Source: CAD feature listing. Evaluate the final solid. Frame: model axes, mm. Face numbers are marked on the shaded views. Coordinates: 2 decimals unless noted, no trailing zeros. Loops run counter-clockwise (first coordinate to the right, second up) from the corner with the lowest first, then second, coordinate; pieces in that order, holes last. Notation, with made-up numbers: (-24.5, 32) -> (30.5, 32) arc R16 cw to (30.5, 62) -> close; hole circle Ø6 at (30.5, -20). An arc over 180 degrees is marked (long way). One line per question, with ' | ' between items. Start each with the question number.
```python
from build123d import *

# Parameters (mm, degrees)
ESQUISSE1_R             = 11
BOSS_EXTRU_1_DEPTH      = 20
ESQUISSE2_R             = 2
ENL_V_MAT_EXTRU_1_DEPTH = 163.249807396


with BuildPart() as part:
    # Esquisse1 → Boss.-Extru.1 (new body)
    with BuildSketch(Plane.XY):
        with BuildLine():
            Line((0, 0), (95, 0))
            Line((95, 0), (74, 108))
            ThreePointArc((74, 108), (47.5, 130), (21, 108))
            Line((21, 108), (0, 0))
        make_face()
        with Locations((47.5, 103.039772727)):
            Circle(ESQUISSE1_R, mode=Mode.SUBTRACT)
    extrude(amount=BOSS_EXTRU_1_DEPTH)

    # Esquisse2 → Enlèv. mat.-Extru.1 (cut, through all)
    with BuildSketch(Plane.XY.offset(20)):
        with Locations((63, 11)):
            Circle(ESQUISSE2_R)
        with Locations((32, 11)):
            Circle(ESQUISSE2_R)
        with Locations((32, 42)):
            Circle(ESQUISSE2_R)
        with Locations((63, 42)):
            Circle(ESQUISSE2_R)
    extrude(amount=-ENL_V_MAT_EXTRU_1_DEPTH, mode=Mode.SUBTRACT)


solid = part.part
```
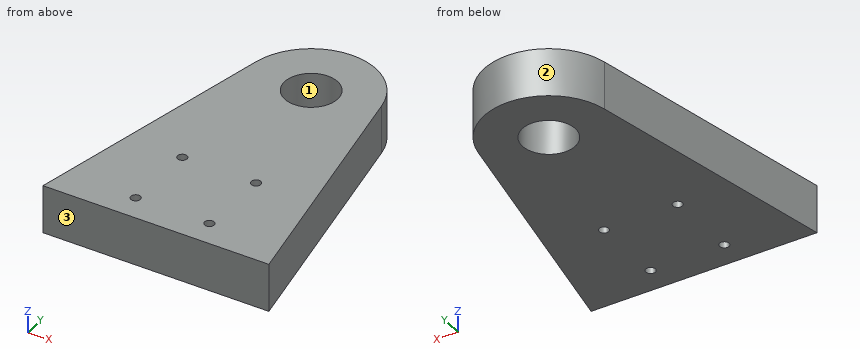
(1) Cut plane D-D, the plane x = 56.5. Return the cut outline in (y, z), and give its area (3 significant figures).
(2) Draft query along Y for the marked faces 1, 2 and 3. Return one class per face: pulls with the +Y half, pulls with the -Y half, needs draft (parallel to the pull), parting line crosses it, or undercut.
(3) Cut plane A-A, the plane y = 42. Return the cut outline in (x, z).
(4) Ray query, L1, parallel to Y at x = 47.5, z = 12; L2, parallel to Y at x = 32, z = 14.5; L3, parallel to X at y = 43.5, z = 1. Return the intervals inside material, ascending.
(5) Cut plane C-C, the plane z = 4. Return the cut outline in (x, y), and give its area (3 significant figures).
(6) Contact query for flat-ended pins moving along their axis: pin 1 Ø3 at (x, z) = (52, 5.5) entering from -Y; pin 2 Ø6 at (x, z) = (23, 15.5) entering from +Y; pin 3 Ø10 at (y, z) = (112.5, 12.5) entering from -X; pin 4 Ø1 at (y, z) = (21, 7.5) entering from -X. Output: stop coordinate, or through.
(7) Cut plane B-B, the plane x = 32. Return the cut outline in (y, z).
Here are the results:
1) outline: (0, 0) -> (96.72, 0) -> (96.72, 20) -> (0, 20) -> close; (109.36, 0) -> (128.45, 0) -> (128.45, 20) -> (109.36, 20) -> close | area: 2,320 mm2
2) face 1: undercut | face 2: pulls with the +Y half | face 3: pulls with the -Y half
3) outline: (8.17, 0) -> (30, 0) -> (30, 20) -> (8.17, 20) -> close; (34, 0) -> (61, 0) -> (61, 20) -> (34, 20) -> close; (65, 0) -> (86.83, 0) -> (86.83, 20) -> (65, 20) -> close
4) L1: y = 0 to 92.04, 114.04 to 130 | L2: y = 0 to 9, 13 to 40, 44 to 125.1 | L3: x = 8.46 to 30.68, 33.32 to 61.68, 64.32 to 86.54
5) outline: (0, 0) -> (95, 0) -> (74, 108) arc R26.96 ccw to (21, 108) -> close; hole circle Ø4 at (32, 11); hole circle Ø4 at (32, 42); hole circle Ø22 at (47.5, 103.04); hole circle Ø4 at (63, 11); hole circle Ø4 at (63, 42) | area: 8,440 mm2
6) pin 1: stops at y = 0 | pin 2: stops at y = 119.31 | pin 3: stops at x = 20.9 | pin 4: stops at x = 3.99
7) outline: (0, 0) -> (9, 0) -> (9, 20) -> (0, 20) -> close; (13, 0) -> (40, 0) -> (40, 20) -> (13, 20) -> close; (44, 0) -> (125.1, 0) -> (125.1, 20) -> (44, 20) -> close
